CAD build for the part. Positions are in the model's coordinates, mm. Give positions to 0.01 mm unless a question says otherwise; leave off trailing zeros. Loops run counter-clockwise (first coordinate to the right, second up) from the corner with the lowest first, then second, coordinate; pieces in that order, holes last.
Item 1: Drop a flat-ended pin along its axis: P1, Ø5, axis at x = 18.5, y = 46.5, coming from the -Z side. Give the stop position or say it passes through.
Item 2: Saw through at B-B on y = 12.7. Give the cut face in (x, z) (3 decimals), plus the area to 3 significant figures.
Item 3: Saw through at C-C on z = 1.2. Give the cut face in (x, y), plus the area to 3 significant figures.
Item 4: Saw through at D-D on y = 64.5. Give the cut face in (x, z) (3 decimals).
Item 5: Saw through at A-A on x = 38.1. Give the cut face in (y, z) (3 decimals).
Item 6: Probe probe 1 along Y at (x, z) = (12.7, 2.5); probe 2 along Y at (x, z) = (11, 1); probe 3 along Y at (x, z) = (38.1, 0.75). List the from-to ranges inside material, lowest first.
Item 7: Mould opens along Y. For faces 1 (the flat face through (39, 76.2, 2)), 2 (the cylindrical face through (13.8, 35.99, 1.61)), 3 (the flat face through (13, 0, 2)), 4 (the flat face through (76.2, 63, 2)) say: released by +Y, released by -Y, zero draft, split by the parting line, or undercut.
Autodesk Inventor part; units mm, degrees
ref_plane "YZ Plane" through (0, 0, 0) normal (1, 0, 0) x (0, 1, 0)
ref_plane "XZ Plane" through (0, 0, 0) normal (0, 1, 0) x (-1, 0, 0)
ref_plane "XY Plane" through (0, 0, 0) normal (0, 0, 1) x (1, 0, 0)
sketch "Sketch1" plane through (0, 0, 0) normal (0, 0, 1) x (1, 0, 0)
  line L0 (0, 0) -> (25.4, 0)
  line L1 (25.4, 0) -> (76.2, 50.8)
  line L2 (76.2, 50.8) -> (76.2, 76.2)
  line L3 (76.2, 76.2) -> (0, 76.2)
  line L4 (0, 76.2) -> (0, 0)
  dimension "d0" = 76.2
  dimension "d1" = 76.2
  dimension "d2" = 25.4
  dimension "d3" = 25.4
extrude "Extrusion1" add sketch "Sketch1" along normal blind 3.175
sketch "Sketch2" plane through (0, 0, 3.175) normal (0, 0, 1) x (1, 0, 0)
  line L0 (0, 0) -> (0, 76.2)
  line L1 (0, 76.2) -> (76.2, 76.2)
  circle A0 centre (12.7, 63.5) radius 2.3813
  dimension "d6" = 4.7625
  dimension "d7" = 12.7
  dimension "d8" = 12.7
extrude "Extrusion2" cut sketch "Sketch2" against normal up to next
pattern_linear "Rectangular Pattern1" count 4 spacing 25.4 along (1, 0, 0) of "Extrusion2"
pattern_linear "Rectangular Pattern2" count 4 spacing 25.4 along (0, -1, 0) of "Extrusion2"
properties part number "Frame_VerticalAngle_Plate" material "Aluminum-6061"
Results below:
1. P1: stops at z = 0
2. outline: (0, 0) - (10.319, 0) - (10.319, 3.175) - (0, 3.175) - close; (15.081, 0) - (38.1, 0) - (38.1, 3.175) - (15.081, 3.175) - close
2. area: 106 mm2
3. outline: (0, 0) - (25.4, 0) - (76.2, 50.8) - (76.2, 76.2) - (0, 76.2) - close; hole circle Ø4.76 at (12.7, 12.7); hole circle Ø4.76 at (12.7, 38.1); hole circle Ø4.76 at (12.7, 63.5); hole circle Ø4.76 at (38.1, 63.5); hole circle Ø4.76 at (63.5, 63.5)
3. area: 4,430 mm2
4. outline: (0, 0) - (10.539, 0) - (10.539, 3.175) - (0, 3.175) - close; (14.861, 0) - (35.939, 0) - (35.939, 3.175) - (14.861, 3.175) - close; (40.261, 0) - (61.339, 0) - (61.339, 3.175) - (40.261, 3.175) - close; (65.661, 0) - (76.2, 0) - (76.2, 3.175) - (65.661, 3.175) - close
5. outline: (12.7, 0) - (61.119, 0) - (61.119, 3.175) - (12.7, 3.175) - close; (65.881, 0) - (76.2, 0) - (76.2, 3.175) - (65.881, 3.175) - close
6. probe 1: y = 0 to 10.32, 15.08 to 35.72, 40.48 to 61.12, 65.88 to 76.2
6. probe 2: y = 0 to 11.03, 14.37 to 36.43, 39.77 to 61.83, 65.17 to 76.2
6. probe 3: y = 12.7 to 61.12, 65.88 to 76.2
7. face 1: released by +Y
7. face 2: undercut
7. face 3: released by -Y
7. face 4: zero draft
